```python
from build123d import *

# Parameters (mm, degrees)
PLATE_SKETCH_W               = 44
PLATE_SKETCH_H               = 15
PLATE_DEPTH                  = 8
TAPPED_HOLE_FACE_D           = 4
TAPPED_HOLE_FACE_CSINK_D     = 4.6
TAPPED_HOLE_FACE_CSINK_ANGLE = 90
RODS_DEPTH                   = 60
RODS_DEPTH_BACK              = 17
RODS_SKETCH_R                = 3
PISTON_SKETCH_R              = 4
PISTON_DEPTH                 = 1
TAPPED_HOLES_TOP_AT_2_COUNT  = 2
TAPPED_HOLES_TOP_AT_2_PITCH  = 35
SHCS_SEAT_SKETCH_R           = 2.75
SHCS_SEAT_DEPTH              = 2.7
SHCS_HEAD_SKETCH_R           = 2.25
SHCS_HEAD_DEPTH              = 2.5
SHCS_HEX_DEPTH               = 1.25
SHCS_CHAM_SIZE               = 0.25
SS_SEAT_SKETCH_R             = 1.5
SS_SEAT_DEPTH                = 2
SS_HEX_DEPTH                 = 1.5


with BuildPart() as part:
    # Plate_Sketch → Plate (new body)
    with BuildSketch(Plane(origin=(0, 0, 0), x_dir=(0, 0, -1), z_dir=(1, 0, 0))):
        Rectangle(PLATE_SKETCH_W, PLATE_SKETCH_H)
    extrude(amount=PLATE_DEPTH)

    # Tapped Hole Face (through all)
    with Locations(Plane(origin=(8, 0, 0), x_dir=(0, 0, -1), z_dir=(1, 0, 0))):
        with Locations((-17.5, 0), (17.5, 0)):
            CounterSinkHole(TAPPED_HOLE_FACE_D / 2, TAPPED_HOLE_FACE_CSINK_D / 2, counter_sink_angle=TAPPED_HOLE_FACE_CSINK_ANGLE)

    # Rods_Sketch → Rods (add, two sides: drawn at the far end of the back side and taken through both)
    with BuildSketch(Plane.ZY.offset(9).offset(-RODS_DEPTH_BACK)):
        with Locations((-10, -1.5)):
            Circle(RODS_SKETCH_R)
        with Locations(Location((10, -1.5, 0), (0, 0, 180))):
            Circle(RODS_SKETCH_R)
    extrude(amount=RODS_DEPTH + RODS_DEPTH_BACK)

    # Piston_Sketch → Piston (add)
    with BuildSketch(Plane.ZY.offset(69)):
        with Locations((-10, -1.5)):
            Circle(PISTON_SKETCH_R)
        with Locations((10, -1.5)):
            Circle(PISTON_SKETCH_R)
    extrude(amount=PISTON_DEPTH)

    # Tapped Holes Top Profile → Tapped Holes Top (revolve, cut)
    with BuildSketch(Plane(origin=(4, 7.5, -17.5), x_dir=(0, 0, 1), z_dir=(1, 0, 0))):
        Polygon((0, 0), (0, 5.420408726), (1.25, 5.2), (1.25, 5), (1.5, 5), (1.5, 0.3), (1.8, 0), align=None)
    tapped_holes_top = revolve(axis=Axis((4, 13.85, -17.5), (0, -1, 0)), mode=Mode.SUBTRACT)

    # Tapped Holes Top at 2: Tapped Holes Top ×2
    with Locations(*[(0, 0, i * TAPPED_HOLES_TOP_AT_2_PITCH) for i in range(1, TAPPED_HOLES_TOP_AT_2_COUNT)]):
        add(tapped_holes_top, mode=Mode.SUBTRACT)

    # Tapped Holes Top Mirror: Tapped Holes Top across plane
    add(tapped_holes_top.mirror(Plane.ZX), mode=Mode.SUBTRACT)

    # Tapped Holes Top Mirror copy 1 sketch → Tapped Holes Top Mirror copy 1 (revolve, cut)
    with BuildSketch(Plane(origin=(4, -7.5, 17.5), x_dir=(0, 0, 1), z_dir=(1, 0, 0))):
        Polygon((0, 0), (0, -5.420408726), (1.25, -5.2), (1.25, -5), (1.5, -5), (1.5, -0.3), (1.8, 0), align=None)
    revolve(axis=Axis((4, -13.85, 17.5), (0, -1, 0)), mode=Mode.SUBTRACT)

    # SHCS Seat_Sketch → SHCS Seat (cut)
    with BuildSketch(Plane(origin=(8, 0, 0), x_dir=(0, 0, -1), z_dir=(1, 0, 0))):
        with Locations((10, -1.5)):
            Circle(SHCS_SEAT_SKETCH_R)
    extrude(amount=-SHCS_SEAT_DEPTH, mode=Mode.SUBTRACT)

    # SHCS Head_Sketch → SHCS Head (add)
    with BuildSketch(Plane(origin=(5.3, 0, 0), x_dir=(0, 0, -1), z_dir=(1, 0, 0))):
        with Locations((10, -1.5)):
            Circle(SHCS_HEAD_SKETCH_R)
    extrude(amount=SHCS_HEAD_DEPTH)

    # SHCS Hex_Sketch → SHCS Hex (cut)
    with BuildSketch(Plane(origin=(7.8, 0, 0), x_dir=(0, 0, -1), z_dir=(1, 0, 0))):
        Polygon((10.577350269, -2.5), (11.154700538, -1.5), (10.577350269, -0.5), (9.422649731, -0.5), (8.845299462, -1.5), (9.422649731, -2.5), align=None)
    extrude(amount=-SHCS_HEX_DEPTH, mode=Mode.SUBTRACT)

    # SHCS Cham
    shcs_cham_edges = [part.edges().sort_by_distance(p)[0] for p in [
        (7.8, -1.5, -7.75),
    ]]
    chamfer(shcs_cham_edges, length=SHCS_CHAM_SIZE)

    # SS Seat_Sketch → SS Seat (cut)
    with BuildSketch(Plane(origin=(0, 7.5, 0), x_dir=(-1, 0, 0), z_dir=(0, 1, 0))):
        with Locations(Location((-4, 10, 0), (0, 0, 90))):
            Circle(SS_SEAT_SKETCH_R)
    extrude(amount=-SS_SEAT_DEPTH, mode=Mode.SUBTRACT)

    # SS Hex_Sketch → SS Hex (cut)
    with BuildSketch(Plane(origin=(0, 5.5, 0), x_dir=(-1, 0, 0), z_dir=(0, 1, 0))):
        Polygon((-4.75, 9.566987298), (-4, 9.133974596), (-3.25, 9.566987298), (-3.25, 10.433012702), (-4, 10.866025404), (-4.75, 10.433012702), align=None)
    extrude(amount=-SS_HEX_DEPTH, mode=Mode.SUBTRACT)


solid = part.part
```
Here's how the part is built. I have some questions about the finished solid (model axes, mm). A direction names the side the tool comes from. Round coordinates to 2 decimals unless told otherwise and drop trailing zeros. Write each loop counter-clockwise with the first axis right and the second up, starting at its lowest first coordinate (ties: lowest second). Pieces come first, ordered by that corner, then holes.
Q1. If we section it at C-C on z = -5: Write out the boundary of the cut face in (x, y).
Q2. Please list where these lines run through material, in increasing order: probe 1 along Z at (x, y) = (4, 4.05); probe 2 along X at (y, z) = (-4, -13); probe 3 along X at (y, z) = (5.9, 17.5).
Q3. If we mould it in two halves opening along Y, with no side actions, what happens to faces 1 (the cylindrical face through (-34, -3.3, -12.4)), 2 (the flat face through (8, 0, 0)), 3 (the cylindrical face through (6.409, -1.401, -7.752)), 4 (the cylindrical face through (3.8, -1.2, -19.1))? For each: +Y half, -Y half, draft (parallel to the pull), parting line (faces both ways), or undercut.
Q4. If we section it at A-A on y = 3.25: Write out the boundary of the cut face in (x, z), plus the area to 3 significant figures.
Q5. Will these pins go through, and if not, where does the flat tip stop? P1, Ø4.5, axis at y = -1.5, z = -10, coming from the +X side; P2, Ø5, axis at x = -3.5, z = -15, coming from the -Y side; P3, Ø2, axis at x = 4, z = -17.5, coming from the +Y side; P4, Ø4, axis at x = 4, z = -17.5, coming from the -Y side.
Q6. Which directions (+Z, -Z, +X, -X, +Y, -Y) give clear straight access to the entire face, cutting with the end or side of a thin tool? Please do faces 5 (the cylindrical face through (4, -5, 16)), 6 (the flat face through (-69, 0, 7)), 7 (the flat face through (-70, -1, 10)), 8 (the cylindrical face through (4, 5, -19)), 9 (the flat face through (4, -7.5, 0)).
Q7. If we section it at B-B on x = -10: Write out the boundary of the cut face in (y, z).
Answer below:
1. outline: (0, -7.5) - (8, -7.5) - (8, 7.5) - (0, 7.5) - close
2. probe 1: z = -22 to -19, -16 to 9.13, 10.87 to 16, 19 to 22
2. probe 2: x = -70 to -69, 0 to 8
2. probe 3: x = 0 to 2.5, 5.5 to 8
3. face 1: parting line
3. face 2: draft
3. face 3: undercut
3. face 4: undercut
4. outline: (0, -22) - (8, -22) - (8, 22) - (0, 22) - close; hole circle Ø3 at (4, -17.5); hole circle Ø3 at (4, 17.5)
4. area: 338 mm2
5. P1: stops at x = 7.8
5. P2: stops at y = -3.16
5. P3: stops at y = 2.26
5. P4: stops at y = -7.5
6. face 5: -Y
6. face 6: none
6. face 7: +Z, -Z, -X, +Y, -Y
6. face 8: +Y
6. face 9: +Z, -Z, +X, -X, -Y
7. outline: circle Ø6 at (-1.5, -10); circle Ø6 at (-1.5, 10)
